Solid Edge part; units mm, degrees
sketch "Sketch1" plane through (0, 0, 0) normal (0, 0, 1) x (1, 0, 0)
  line L0 (-100, 100) -> (-100, -100)
  line L1 (-100, -100) -> (100, -100)
  line L2 (100, -100) -> (100, 100)
  line L3 (100, 100) -> (-100, 100)
extrude "Protrusion1" add sketch "Sketch1" along normal blind 40
sketch "Sketch2" plane through (0, 0, 0) normal (0, 0, 1) x (1, 0, 0)
  line L0 (-97.8, 97.8) -> (-97.8, -97.8)
  line L1 (-97.8, -97.8) -> (97.8, -97.8)
  line L2 (97.8, -97.8) -> (97.8, 97.8)
  line L3 (97.8, 97.8) -> (-97.8, 97.8)
extrude "ExtrudedCutout_1" cut sketch "Sketch2" along normal blind 45
sketch "Sketch3" plane through (0, 0, 0) normal (0, 0, 1) x (1, 0, 0)
  line L0 (-100, -100) -> (100, -100)
  line L1 (100, -100) -> (100, 100)
  line L2 (100, 100) -> (-100, 100)
  line L3 (-100, 100) -> (-100, -100)
extrude "Boden" add sketch "Sketch3" against normal blind 2
sketch "Sketch4" plane through (0, 0, 40) normal (0, 0, 1) x (0, -1, 0)
  line L0 (-97.8, -97.8) -> (-97.8, 97.8)
  line L1 (-97.8, 97.8) -> (97.8, 97.8)
  line L2 (97.8, 97.8) -> (97.8, -97.8)
  line L3 (97.8, -97.8) -> (-97.8, -97.8)
  line L4 (-100, -100) -> (-100, 100)
  line L5 (-100, 100) -> (100, 100)
  line L6 (100, 100) -> (100, -100)
  line L7 (100, -100) -> (-100, -100)
extrude "Verbindung" add sketch "Sketch4" along normal blind 2
sketch "Sketch5" plane through (0, 0, 40) normal (0, 0, 1) x (0, -1, 0)
  line L0 (-96, 96) -> (-96, -96)
  line L1 (-96, -96) -> (96, -96)
  line L2 (96, -96) -> (96, 96)
  line L3 (96, 96) -> (-96, 96)
  line L4 (-97.8, -97.8) -> (-97.8, 97.8)
  line L5 (-97.8, 97.8) -> (97.8, 97.8)
  line L6 (97.8, 97.8) -> (97.8, -97.8)
  line L7 (97.8, -97.8) -> (-97.8, -97.8)
extrude "ExtrudedProtrusion_7" add sketch "Sketch5" along normal blind 7
fillet "Round_1" radius 1 1 edges at (97.8, 0, 40)
fillet "Round_2" radius 1 9 edges at (-0.5, -97.8, 40) (97.5071, -97.8, 39.7071) (97.8, -97.8, 19.5) (-97.8, 0, 40) (-97.8, -97.8, 20) (-0.5, 97.8, 40) (97.5071, 97.8, 39.7071) (97.8, 97.8, 19.5) (-97.8, 97.8, 20)
Model file for the job. Use its own axes, mm. A direction names the side the tool comes from. Coordinates: 2 decimals unless noted, no trailing zeros. Loops run counter-clockwise (first coordinate to the right, second up) from the corner with the lowest first, then second, coordinate; pieces in that order, holes last. Notation, with made-up numbers: (-34, 79.25) - (17, 79.25) arc R25 ccw to (17, 95.25) - close; hole circle Ø4 at (15, 42). An arc over 180 degrees is marked (long way). Answer as a JSON object with one key per item and string values. Group by question number.
(1) Cut at B-B (x = -61.5). Give the cut face in (y, z), then the cut area to 3 significant figures.
(2) Two-plate mould, pull along Z, no slides. Class faces 6 (the face through (96, -1, 43)), 7 (the face through (-1, 1, -2)), 8 (the face through (-1, 97.8, 19)): released by +Z, released by -Z, zero draft, split by the parting line, or undercut.
(3) Cut at A-A (z = 31.5). Give the cut face in (x, y), then the cut area to 3 significant figures.
(4) Tool access for faces 1 (the face through (97.8, 1, 44)), 2 (the face through (-1, -96, 43)), 3 (the face through (1, -97.8, 19)), 4 (the face through (1, -97.8, 44)), 5 (the face through (100, -1, 20)): list every direction of +Z, -Z, +X, -X, +Y, -Y with a clear straight run to the whole face (end or side of a thin tool).
(5) Probe line 1 along Y through (x, z) = (-66, 6.5); line 2 along X through (y, z) = (-3.5, 39.5). List the from-to ranges inside material, lowest first.
(6) Flat gauge pins, fed straight in: pin 1 (12 mm diameter, centred on x = -29, y = 6, fed in from +Z); pin 2 (4 mm diameter, centred on x = -15.5, z = 45.5, fed in from +Y); pin 3 (1.5 mm diameter, centred on x = 39, z = 44, fed in from -Y). Where does each tip first touch, or does it go through?
Geometry says:
{
 "1": {"outline": "(-100, -2) - (100, -2) - (100, 42) - (97.8, 42) - (97.8, 47) - (96, 47) - (96, 40) - (96.8, 40) arc R1 cw to (97.8, 39) - (97.8, 0) - (-97.8, 0) - (-97.8, 39) arc R1 cw to (-96.8, 40) - (-96, 40) - (-96, 47) - (-97.8, 47) - (-97.8, 42) - (-100, 42) - close", "area": "610 mm^2"},
 "2": {"face 6": "zero draft", "face 7": "released by -Z", "face 8": "undercut"},
 "3": {"outline": "(-100, -100) - (100, -100) - (100, 100) - (-100, 100) - close; hole (-97.8, -96.8) arc R1 ccw to (-96.8, -97.8) - (96.8, -97.8) arc R1 ccw to (97.8, -96.8) - (97.8, 96.8) arc R1 ccw to (96.8, 97.8) - (-96.8, 97.8) arc R1 ccw to (-97.8, 96.8) - close", "area": "1,740 mm^2"},
 "4": {"face 1": "+Z, +X, +Y, -Y", "face 2": "+Z", "face 3": "none", "face 4": "+Z, +X, -X, -Y", "face 5": "+Z, -Z, +X, +Y, -Y"},
 "5": {"line 1": "y = -100 to -97.8, 97.8 to 100", "line 2": "x = -100 to -97.67, 97.67 to 100"},
 "6": {"pin 1": "stops at z = 0", "pin 2": "stops at y = 97.8", "pin 3": "stops at y = -97.8"}
}
